Autodesk Inventor part; units mm, degrees
ref_plane "YZ Plane" through (0, 0, 0) normal (1, 0, 0) x (0, 1, 0)
ref_plane "XZ Plane" through (0, 0, 0) normal (0, 1, 0) x (-1, 0, 0)
ref_plane "XY Plane" through (0, 0, 0) normal (0, 0, 1) x (1, 0, 0)
sketch "スケッチ1" plane through (0, 0, 0) normal (0, 0, 1) x (1, 0, 0)
  circle A0 centre (0, 0) radius 10
  circle A1 centre (0, 0) radius 2
  dimension "d0" = 20
  dimension "d1" = 4
extrude "押し出し1" add sketch "スケッチ1" along normal blind 3
sketch "スケッチ2" plane through (0, 0, 3) normal (0, 0, 1) x (1, 0, 0)
  circle A0 centre (0, 0) radius 5.5
  circle A1 centre (-5.5, 0) radius 1.7
  circle A2 centre (5.5, 0) radius 1.7
  dimension "d4" = 11
  dimension "d5" = 3.4
  dimension "d6" = 3.4
extrude "押し出し2" cut sketch "スケッチ2" against normal blind 3 contours A0 A2 | A0 A2 | A1 A0 | A0 A1
fillet "フィレット1" radius 0.3 2 edges at (-10, 0, 3) (-10, 0, 0)
properties part number "homemade_setcolor" material "アルミニウム 6061"
Verification items for the finished model (mm, model axes). Coordinates: 2 decimals unless noted, no trailing zeros. Write each loop counter-clockwise with the first axis right and the second up, starting at its lowest first coordinate (ties: lowest second). Pieces come first, ordered by that corner, then holes. Notation, with made-up numbers: (14, 85.25) - (35, 85.25) arc R22 ccw to (35, 120.25) - close; hole circle Ø3 at (79.25, 19.25). An arc over 180 degrees is marked (long way). One line per question, with ' | ' between items. Start each with the question number.
1. Section check B-B (y = 0). Enter the section's corners in (x, z).
2. Material ranges on line 1 along Y through (x, z) = (0, 1.3); line 2 along X through (y, z) = (-1, 2.4); line 3 along Y through (x, z) = (-6.5, 1.35), recorded low to high.
3. Section check A-A (x = 0). Enter the section's corners in (y, z).
4. Section check C-C (z = 0.75). Enter the section's corners in (x, y), plus the area to 3 significant figures.
5. Gauge pin test, flat ends, axial feed: P1, Ø1, axis at x = -7, y = -0.5, coming from the +Z side; P2, Ø1, axis at y = 4, z = 2, coming from the +X side; P3, Ø1, axis at y = 3, z = 0.5, coming from the +X side. Record the tip position at first contact, or that the pin passes through.
6. Draft check along X on faces 1 (the cylindrical face through (-2.17, 9.76, 1.48)), 2 (the flat face through (-0.1, 2.3, 3)), 3 (the cylindrical face through (0, 2, 1)). Enter one of: released by +X, released by -X, zero draft, split by the parting line, or undercut.
Computed values:
1) outline: (-10, 0.3) arc R0.3 ccw to (-9.7, 0) - (-7.2, 0) - (-7.2, 3) - (-9.7, 3) arc R0.3 ccw to (-10, 2.7) - close; (-3.8, 0) - (-2, 0) - (-2, 3) - (-3.8, 3) - close; (2, 0) - (3.8, 0) - (3.8, 3) - (2, 3) - close; (7.2, 0) - (9.7, 0) arc R0.3 ccw to (10, 0.3) - (10, 2.7) arc R0.3 ccw to (9.7, 3) - (7.2, 3) - close
2) line 1: -10 to -2, 2 to 10 | line 2: -9.95 to -6.87, -4.13 to -1.73, 1.73 to 4.13, 6.87 to 9.95 | line 3: -7.6 to -1.37, 1.37 to 7.6
3) outline: (-10, 0.3) arc R0.3 ccw to (-9.7, 0) - (-2, 0) - (-2, 3) - (-9.7, 3) arc R0.3 ccw to (-10, 2.7) - close; (2, 0) - (9.7, 0) arc R0.3 ccw to (10, 0.3) - (10, 2.7) arc R0.3 ccw to (9.7, 3) - (2, 3) - close
4) outline: circle Ø20 at (0, 0); hole circle Ø3.4 at (-5.5, 0); hole circle Ø4 at (0, 0); hole circle Ø3.4 at (5.5, 0) | area: 283 mm²
5) P1: z = 3 | P2: x = 9.37 | P3: x = 9.68
6) face 1: split by the parting line | face 2: zero draft | face 3: undercut
